Read the model definition and answer for the solid it produces. Units are mm, in the model's axes. Give positions to 0.01 mm unless a question says otherwise; leave off trailing zeros. Write each loop counter-clockwise with the first axis right and the second up, starting at its lowest first coordinate (ties: lowest second). Pieces come first, ordered by that corner, then holes.
```python
from build123d import *

# Parameters (mm, degrees)
CYLINDER004_R     = 3.5
CYLINDER004_DEPTH = 10
BOX004_W          = 10
BOX004_H          = 110
BOX004_DEPTH      = 10
CYLINDER003_R     = 10
CYLINDER003_DEPTH = 1.5
BOX002_W          = 1.5
BOX002_H          = 170
BOX002_DEPTH      = 20
CYLINDER002_R     = 10
CYLINDER002_DEPTH = 1.5


with BuildPart() as pwrjack:
    # Cylinder004 → Cylinder004 (new body)
    with BuildSketch(Plane(origin=(-3, 9, 0), x_dir=(0, 0, -1), z_dir=(1, 0, 0))):
        Circle(CYLINDER004_R)
    extrude(amount=CYLINDER004_DEPTH)


with BuildPart() as cube003:
    # Box004 → Box004 (new body)
    with BuildSketch(Plane(origin=(-3, 38, -5), x_dir=(1, 0, 0), z_dir=(0, 0, 1))):
        with Locations((5, 55)):
            Rectangle(BOX004_W, BOX004_H)
    extrude(amount=BOX004_DEPTH)


with BuildPart() as cylinder003:
    # Cylinder003 → Cylinder003 (new body)
    with BuildSketch(Plane(origin=(0, 169, 0), x_dir=(0, 0, -1), z_dir=(1, 0, 0))):
        Circle(CYLINDER003_R)
    extrude(amount=CYLINDER003_DEPTH)


with BuildPart() as cube002:
    # Box002 → Box002 (new body)
    with BuildSketch(Plane.XY.offset(-10)):
        with Locations((0.75, 85)):
            Rectangle(BOX002_W, BOX002_H)
    extrude(amount=BOX002_DEPTH)


with BuildPart() as cut003:
    # Cylinder002 → Cylinder002 (new body)
    with BuildSketch(Plane(origin=(0, 0, 0), x_dir=(0, 0, -1), z_dir=(1, 0, 0))):
        Circle(CYLINDER002_R)
    extrude(amount=CYLINDER002_DEPTH)

    # Fusion001: union Cylinder003, Cube002
    add(cylinder003.part)
    add(cube002.part)

    # Cut001: cut Cube003
    add(cube003.part, mode=Mode.SUBTRACT)

    # Cut003: cut pwrjack
    add(pwrjack.part, mode=Mode.SUBTRACT)


solid = cut003.part
```
Item 1: Section D-D (y = 9) is taken. Write down the section's boundary in (x, z), and give its area (3 significant figures).
Result set:
outline: (0, -10) - (1.5, -10) - (1.5, -3.5) - (0, -3.5) - close; (0, 3.5) - (1.5, 3.5) - (1.5, 10) - (0, 10) - close
area: 19.5 mm2
Item 2: Determine the mould class of faces 1 (the cylindrical face through (1, 179, 0)), 2 (the flat face through (1.5, 86, -7)), 3 (the cylindrical face through (0.74, 5.583, 0.759)) for opening direction Y: pulls with the +Y half, pulls with the -Y half, needs draft (parallel to the pull), parting line crosses it, or undercut.
Result set:
face 1: pulls with the +Y half
face 2: needs draft
face 3: undercut
Item 3: Find the intervals of material crossed by line 1 along Y through (x, z) = (0.35, 0); line 2 along Z through (x, y) = (0.5, 9); line 3 along Z through (x, y) = (1.1, 79), in increasing order.
Result set:
line 1: y = -10 to 5.5, 12.5 to 38, 148 to 179
line 2: z = -10 to -3.5, 3.5 to 10
line 3: z = -10 to -5, 5 to 10
Item 4: Section C-C (z = 0) is taken. Write down the section's boundary in (x, y).
Result set:
outline: (0, -10) - (1.5, -10) - (1.5, 5.5) - (0, 5.5) - close; (0, 12.5) - (1.5, 12.5) - (1.5, 38) - (0, 38) - close; (0, 148) - (1.5, 148) - (1.5, 179) - (0, 179) - close
Item 5: Section B-B (x = 0.7) is taken. Write down the section's boundary in (y, z), and give its area (3 significant figures).
Result set:
outline: (0, -10) - (170, -10) - (170, -9.95) arc R10 ccw to (170, 9.95) - (170, 10) - (0, 10) arc R10 ccw to start; hole circle Ø7 at (9, 0); hole (38, -5) - (148, -5) - (148, 5) - (38, 5) - close
area: 2,560 mm2
Item 6: Section A-A (y = 78) is taken. Write down the section's boundary in (x, z).
Result set:
outline: (0, -10) - (1.5, -10) - (1.5, -5) - (0, -5) - close; (0, 5) - (1.5, 5) - (1.5, 10) - (0, 10) - close
